from build123d import *

# Parameters (mm, degrees)
F0_W     = 48
F0_H     = 63
F0_R     = 2.25
F1_DEPTH = 2


with BuildPart() as f1:
    # F0 (on Front) → F1 (new body)
    with BuildSketch(Plane.XZ):
        Rectangle(F0_W, F0_H)
        with Locations((-19, -26.5)):
            Circle(F0_R, mode=Mode.SUBTRACT)
        with Locations((19, -26.5)):
            Circle(F0_R, mode=Mode.SUBTRACT)
        with BuildLine():
            ThreePointArc((9, -5), (11, -7), (9, -9))
            Line((9, -9), (-9, -9))
            ThreePointArc((-9, -9), (-11, -7), (-9, -5))
            Line((-9, -5), (9, -5))
        make_face(mode=Mode.SUBTRACT)
        with Locations((-19, 26.5)):
            Circle(F0_R, mode=Mode.SUBTRACT)
        with BuildLine():
            Line((-9, 3), (9, 3))
            ThreePointArc((9, 3), (12, 0), (9, -3))
            Line((9, -3), (-9, -3))
            ThreePointArc((-9, -3), (-12, 0), (-9, 3))
        make_face(mode=Mode.SUBTRACT)
        with BuildLine():
            ThreePointArc((9, 9), (11, 7), (9, 5))
            Line((9, 5), (-9, 5))
            ThreePointArc((-9, 5), (-11, 7), (-9, 9))
            Line((-9, 9), (9, 9))
        make_face(mode=Mode.SUBTRACT)
        with Locations((19, 26.5)):
            Circle(F0_R, mode=Mode.SUBTRACT)
    extrude(amount=F1_DEPTH)


solid = f1.part
CAD build for the part. Positions are in the model's coordinates, mm. A direction names the side the tool comes from. Round coordinates to 2 decimals unless told otherwise and drop trailing zeros. Write each loop counter-clockwise with the first axis right and the second up, starting at its lowest first coordinate (ties: lowest second). Pieces come first, ordered by that corner, then holes. Notation, with made-up numbers: M 89,50.25 L 121,50.25 A37 cw 121,87.25 Z; hole C 79,23.25 d11. An arc over 180 degrees is marked long. Use a Markdown table: item, result. Add a question column.
1. 3-axis set-ups, long thin cutter, end or side, ignore diameter. For faces 4 (the face through (0, 0, -14)), 5 (the face through (-12, -1, 0)): which of +Z, -Z, +X, -X, +Y, -Y reach the whole face in a straight line?
2. Pull direction X, two halves, no side cores. Call faces 1 (the face through (20.038, -0.986, -28.496)), 2 (the face through (-24, -1, 0)), 3 (the face through (0, -1, 31.5)): released by +X, released by -X, zero draft, split by the parting line, or undercut.
3. Slice it at C-C on z = -7. Give the cut face in (x, y).
4. Slice it at D-D on x = 19. Give the cut face in (y, z).
5. Drill centre lines: probe 1 along Z at (x, y) = (-19, -1.15); probe 2 along Z at (x, y) = (-1.5, -0.55); probe 3 along Z at (x, y) = (-18, -1.5). Where is each one in solid material? Low to high.
6. Slice it at B-B on y = -0.8. Give the cut face in (x, z).
7. Slice it at A-A on x = 3.5. Give the cut face in (y, z), then the cut area to 3 significant figures.
8. Flat gauge pin, fed straight in: P1, Ø3.5, axis at x = -19, z = 26.5, coming from the +Y side. Where does the tip first touch, or does it go through?
Reply:
| question | item | result |
|---|---|---|
| 1 | face 4 | +Z, -Z, +X, -X, +Y |
| 1 | face 5 | +Y, -Y |
| 2 | face 1 | undercut |
| 2 | face 2 | released by -X |
| 2 | face 3 | zero draft |
| 3 | outline | M -24,-2 L -11,-2 L -11,0 L -24,0 Z; M 11,-2 L 24,-2 L 24,0 L 11,0 Z |
| 4 | outline | M -2,-31.5 L 0,-31.5 L 0,-28.75 L -2,-28.75 Z; M -2,-24.25 L 0,-24.25 L 0,24.25 L -2,24.25 Z; M -2,28.75 L 0,28.75 L 0,31.5 L -2,31.5 Z |
| 5 | probe 1 | z = -31.5 to -28.75, -24.25 to 24.25, 28.75 to 31.5 |
| 5 | probe 2 | z = -31.5 to -9, -5 to -3, 3 to 5, 9 to 31.5 |
| 5 | probe 3 | z = -31.5 to -28.52, -24.48 to 24.48, 28.52 to 31.5 |
| 6 | outline | M -24,-31.5 L 24,-31.5 L 24,31.5 L -24,31.5 Z; hole C -19,-26.5 d4.5; hole C -19,26.5 d4.5; hole M -9,-9 L 9,-9 A2 ccw 9,-5 L -9,-5 A2 ccw Z; hole M -9,-3 L 9,-3 A3 ccw 9,3 L -9,3 A3 ccw Z; hole M -9,5 L 9,5 A2 ccw 9,9 L -9,9 A2 ccw Z; hole C 19,-26.5 d4.5; hole C 19,26.5 d4.5 |
| 7 | outline | M -2,-31.5 L 0,-31.5 L 0,-9 L -2,-9 Z; M -2,-5 L 0,-5 L 0,-3 L -2,-3 Z; M -2,3 L 0,3 L 0,5 L -2,5 Z; M -2,9 L 0,9 L 0,31.5 L -2,31.5 Z |
| 7 | area | 98.0 mm^2 |
| 8 | P1 | passes through |
